Source: three-view drawing plus pictorial views. Frame: mm from the lowest corner of the part. A direction names the side the tool comes from. Give positions to 0.01 mm unless a question says otherwise; leave off trailing zeros. Loops run counter-clockwise (first coordinate to the right, second up) from the corner with the lowest first, then second, coordinate; pieces in that order, holes last.
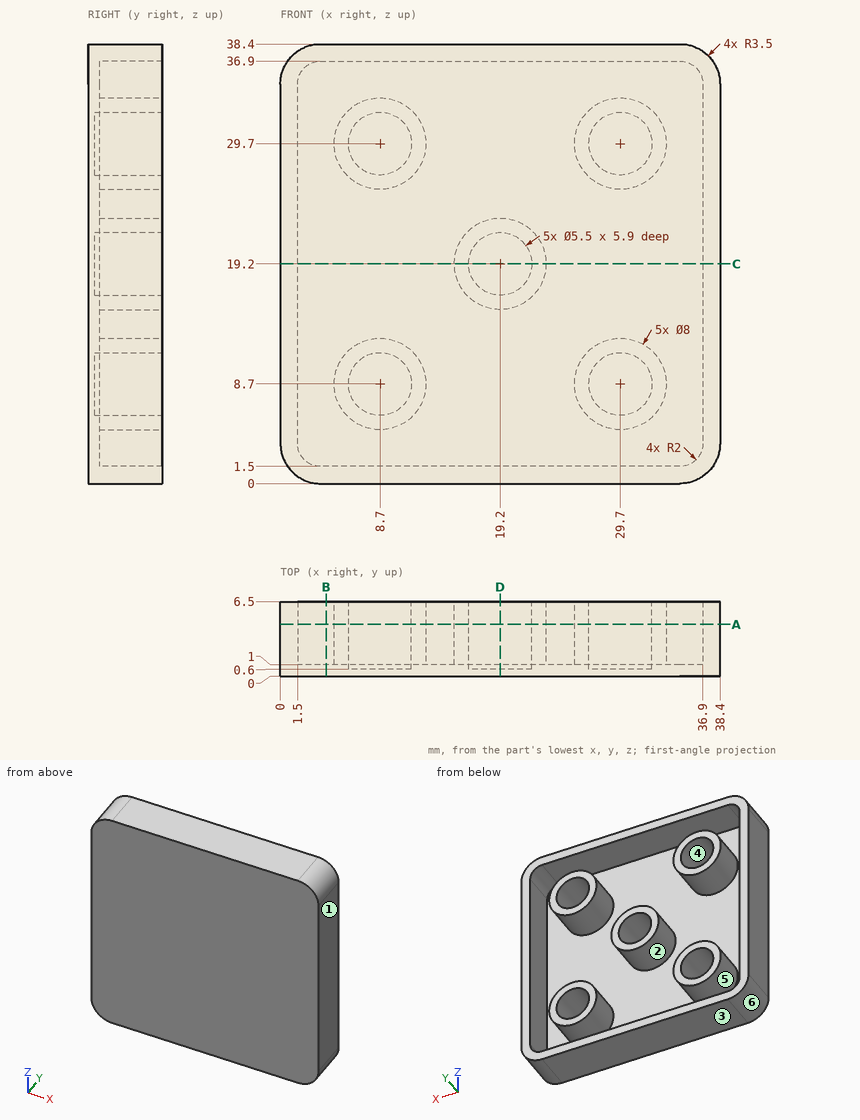
1) Cut plane B-B (x = 4). Return loops of the section in (y, z), and give its area (3 significant figures).
Checks:
outline: (0, 0) - (6.5, 0) - (6.5, 1.5) - (1, 1.5) - (1, 36.9) - (6.5, 36.9) - (6.5, 38.4) - (0, 38.4) - close
area: 54.9 mm2
2) Cut plane D-D (x = 19.2). Return loops of the section in (y, z), and give its area (4 significant figures).
Checks:
outline: (0, 0) - (6.5, 0) - (6.5, 1.5) - (1, 1.5) - (1, 15.2) - (6.5, 15.2) - (6.5, 16.45) - (0.6, 16.45) - (0.6, 21.95) - (6.5, 21.95) - (6.5, 23.2) - (1, 23.2) - (1, 36.9) - (6.5, 36.9) - (6.5, 38.4) - (0, 38.4) - close
area: 66.45 mm2
3) Contact query for flat-ended pins moving along their axis: P1, Ø1.6, axis at x = 10, z = 29, coming from the +Y side; P2, Ø2, axis at x = 19, z = 5.5, coming from the +Y side. Output: stop coordinate, or through.
Checks:
P1: stops at y = 0.6
P2: stops at y = 1
4) Cut plane C-C (z = 19.2). Return loops of the section in (x, y), and give its area (4 significant figures).
Checks:
outline: (0, 0) - (38.4, 0) - (38.4, 6.5) - (36.9, 6.5) - (36.9, 1) - (23.2, 1) - (23.2, 6.5) - (21.95, 6.5) - (21.95, 0.6) - (16.45, 0.6) - (16.45, 6.5) - (15.2, 6.5) - (15.2, 1) - (1.5, 1) - (1.5, 6.5) - (0, 6.5) - close
area: 66.45 mm2
5) Cut plane A-A (y = 4.5). State how many separate pieces and enclosed holes the cut face has, and give its area (3 significant figures).
Checks:
separate pieces: 6
enclosed holes: 6
area: 347 mm2
6) Pull-direction query (X, two-part tool) for the marked faces 1, 2, 3 and 4; classes: released by +X, released by -X, zero draft, split by the parting line, or undercut.
Checks:
face 1: released by +X
face 2: undercut
face 3: zero draft
face 4: undercut
7) Ray query, probe 1 along X at (y, z) = (1.95, 8.7); probe 2 along Z at (x, y) = (19.2, 4). Return the intervals inside material, ascending.
Checks:
probe 1: x = 0 to 1.5, 4.7 to 5.95, 11.45 to 12.7, 25.7 to 26.95, 32.45 to 33.7, 36.9 to 38.4
probe 2: z = 0 to 1.5, 15.2 to 16.45, 21.95 to 23.2, 36.9 to 38.4
8) Reachability of the marked faces 5 and 6 from +Z, -Z, +X, -X, +Y, -Y: full face, straight path, thin tool, end or side. Return the list, or none.
Checks:
face 5: +Y
face 6: -Z, -X, +Y, -Y
